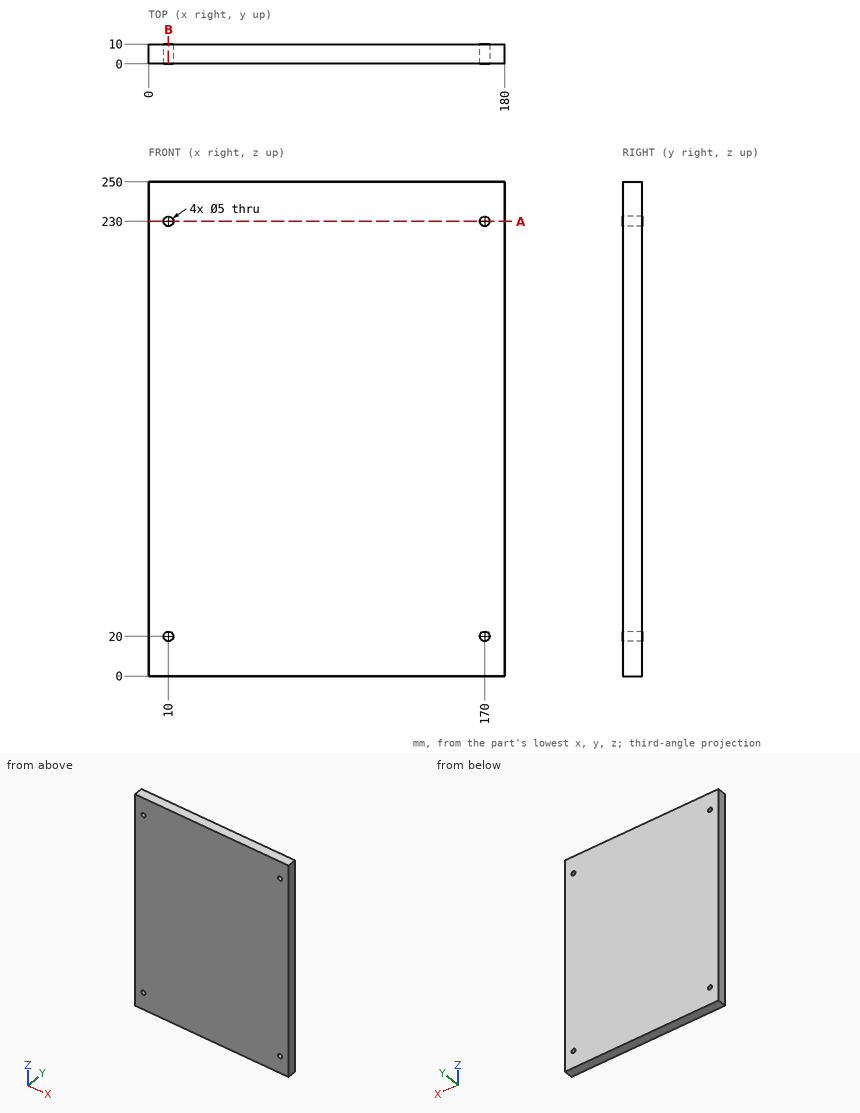
Answer from the drawing. Dimensions are ordinates in mm from the lowest x, y and z of the part. Give positions to 0.01 mm unless a question says otherwise; leave off trailing zeros. Loops run counter-clockwise (first coordinate to the right, second up) from the corner with the lowest first, then second, coordinate; pieces in that order, holes last. Notation, with made-up numbers: (65, 49) - (121, 49) arc R31 cw to (121, 84) - close; hole circle Ø11 at (-39, 52). An arc over 180 degrees is marked (long way). Answer as CSV lines item,"result". Start each with the question number.
Item 1: Find the intervals of material crossed by line 1 (Z direction, x = 170, y = 2); line 2 (X direction, y = 5.75, z = 230), in increasing order. Write a range as from..to.
Item 2: A cutting plane is placed at A-A on z = 230. Determine the outline of the cut face in (x, y), then the cut area to 3 significant figures.
Item 3: A cutting plane is placed at B-B on x = 10. Determine the outline of the cut face in (y, z).
Found:
1,line 1,"z = 0..17.5, 22.5..227.5, 232.5..250"
1,line 2,"x = 0..7.5, 12.5..167.5, 172.5..180"
2,outline,"(0, 0) - (7.5, 0) - (7.5, 10) - (0, 10) - close; (12.5, 0) - (167.5, 0) - (167.5, 10) - (12.5, 10) - close; (172.5, 0) - (180, 0) - (180, 10) - (172.5, 10) - close"
2,area,"1,700 mm^2"
3,outline,"(0, 0) - (10, 0) - (10, 17.5) - (0, 17.5) - close; (0, 22.5) - (10, 22.5) - (10, 227.5) - (0, 227.5) - close; (0, 232.5) - (10, 232.5) - (10, 250) - (0, 250) - close"
